Study the drawing (mm; zero at the part's minimum x, y, z) and answer. A direction names the side the tool comes from. Coordinates: 2 decimals unless noted, no trailing zeros. Loops run counter-clockwise (first coordinate to the right, second up) from the corner with the lowest first, then second, coordinate; pieces in that order, holes last. Notation, with made-up numbers: (-16.5, 63) - (3.5, 63) arc R24 cw to (3.5, 78) - close; hole circle Ø2 at (-38, 18.25). An arc over 180 degrees is marked (long way). Put each result on its own line as item: value.
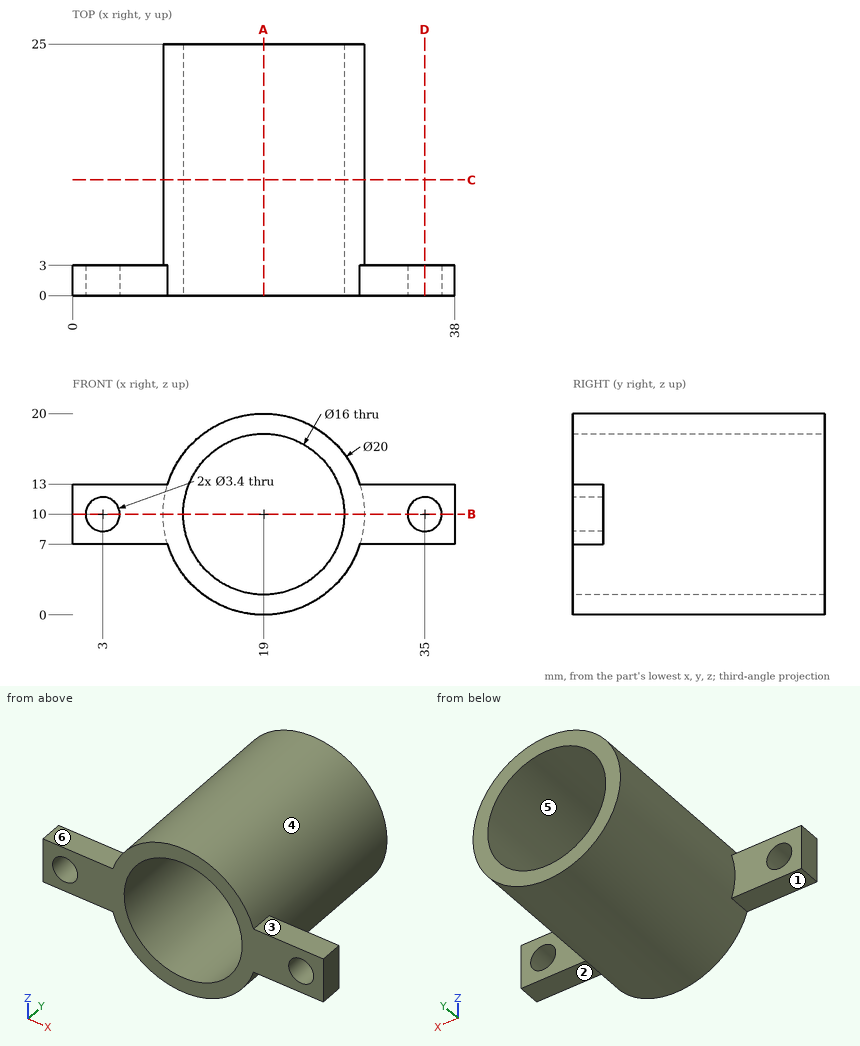
1) For a pull along X with two mould halves and no side action, classify the marked faces 4, 5 and 6 as pulls with the +X half, pulls with the -X half, needs draft (parallel to the pull), parting line crosses it, or undercut.
Found:
face 4: parting line crosses it
face 5: undercut
face 6: needs draft
2) For the marked faces 1, 2 and 3, determine the directions among +Z, -Z, +X, -X, +Y, -Y from which every point of the face is accessible in a straight line to the end or side of a thin tool.
Found:
face 1: -Z, -X, +Y, -Y
face 2: -Z, +X, +Y, -Y
face 3: +Z, +X, +Y, -Y
3) The part is cut by section D-D (x = 35). Give the vertices of the cut face in (y, z).
Found:
outline: (0, 7) - (3, 7) - (3, 8.3) - (0, 8.3) - close; (0, 11.7) - (3, 11.7) - (3, 13) - (0, 13) - close
4) The part is cut by section C-C (y = 11.5). Give the vertices of the cut face in (x, z), and give its area (3 significant figures).
Found:
outline: circle Ø20 at (19, 10); hole circle Ø16 at (19, 10)
area: 113 mm^2
5) The part is cut by section B-B (z = 10). Give the vertices of the cut face in (x, y).
Found:
outline: (0, 0) - (1.3, 0) - (1.3, 3) - (0, 3) - close; (4.7, 0) - (11, 0) - (11, 25) - (9, 25) - (9, 3) - (4.7, 3) - close; (27, 0) - (33.3, 0) - (33.3, 3) - (29, 3) - (29, 25) - (27, 25) - close; (36.7, 0) - (38, 0) - (38, 3) - (36.7, 3) - close
6) The part is cut by section A-A (x = 19). Give the vertices of the cut face in (y, z).
Found:
outline: (0, 0) - (25, 0) - (25, 2) - (0, 2) - close; (0, 18) - (25, 18) - (25, 20) - (0, 20) - close
7) Straight lines are drawn through the part: L1, parallel to X at y = 1.5, z = 10; L2, parallel to Z at x = 3, y = 2.2; L3, parallel to X at y = 10, z = 10. For each, find the intervals that lie inside material, in ascending order. Write a range as [from, to].
Found:
L1: x = [0, 1.3], [4.7, 11], [27, 33.3], [36.7, 38]
L2: z = [7, 8.3], [11.7, 13]
L3: x = [9, 11], [27, 29]
8) Each of these flat-tipped pins is pushed along its axis until it touches: pin 1 (1 mm diameter, centred on y = 8.5, z = 16.5, fed in from -X); pin 2 (5.5 mm diameter, centred on x = 35, z = 10, fed in from +Y); pin 3 (1.5 mm diameter, centred on y = 4.5, z = 14, fed in from -X). Where does it stop, or does it pass through?
Found:
pin 1: stops at x = 11
pin 2: stops at y = 3
pin 3: stops at x = 9.54
